For this review, take the finished solid that the model builds, in its own axes (mm). Face numbers are marked on the shaded views. A direction names the side the tool comes from. Coordinates: 2 decimals unless noted, no trailing zeros. Write each loop counter-clockwise with the first axis right and the second up, starting at its lowest first coordinate (ties: lowest second). Pieces come first, ordered by that corner, then holes. Notation, with made-up numbers: (52, 10) - (87, 10) arc R27 ccw to (87, 46) - close; hole circle Ø6 at (41, 44.25). An arc over 180 degrees is marked (long way). Use one line per item in the form item = value. Start each with the question number.
1) We need section C-C (x = 20). Give the boundary of the cut face in (y, z), plus the area to 3 significant figures.
2) Mouldability with a two-part tool opening along X and no side actions: class the marked faces 1, 2 and 3 as pulls with the +X half, pulls with the -X half, needs draft (parallel to the pull), parting line crosses it, or undercut.
3) We need section B-B (x = -22). Give the boundary of the cut face in (y, z).
4) We need section D-D (y = -24). Give the boundary of the cut face in (x, z), plus the area to 3 significant figures.
5) Tool access review of the marked faces 4 and 5: name each direction out of +Z, -Z, +X, -X, +Y, -Y from which nothing blocks a thin tool from reaching the whole face with its end or side.
6) Insertion check: P1, Ø6, axis at y = 11.5, z = 35, coming from the -X side (3 decimals); P2, Ø10, axis at y = 10, z = 96, coming from the -X side; P3, Ø4.5, axis at x = 0, y = 0, coming from the +Z side; P4, Ø10, axis at x = -18, y = 18, coming from the +Z side. Each pin has a flat end and moves straight along its axis. Give the tip position at first contact, or say it passes through.
7) For L1, parallel to X at y = -4, z = 90.5; L2, parallel to X at y = 0, z = 7.25; L3, parallel to X at y = -34.5, z = 57, list the stretches that pass through material, from the lowest coordinate up. Write a range as from..to.
```python
from build123d import *

# Parameters (mm, degrees)
SKETCH1_R           = 6.35
BOSS_EXTRUDE5_DEPTH = 220
SKETCH9_R           = 10
BOSS_EXTRUDE6_DEPTH = 2.5
SKETCH10_R          = 12.5
BOSS_EXTRUDE7_DEPTH = 2
SKETCH7_R           = 2.54
CUT_EXTRUDE1_DEPTH  = 19
CUT_EXTRUDE2_DEPTH  = 19


with BuildPart() as part:
    # Sketch1 → Boss-Extrude5 (new body)
    with BuildSketch(Plane.XY):
        Circle(SKETCH1_R)
        with BuildLine():
            ThreePointArc((0.744012112, -6.306262441), (0.372648292, -6.33905618), (0, -6.35))
            Line((0, -6.35), (0, -38.1))
            ThreePointArc((0, -38.1), (2.307620454, -36.88268092), (3.706666044, -34.680488981))
            ThreePointArc((3.706666044, -34.680488981), (3.812853299, -34.161384534), (3.809033576, -33.631544397))
            Line((3.809033576, -33.631544397), (0.744012112, -6.306262441))
        make_face()
        with BuildLine():
            ThreePointArc((-5.089377421, -3.79746461), (-5.303459542, -3.492250977), (-5.499261314, -3.175))
            Line((-5.499261314, -3.175), (-32.995567884, -19.05))
            ThreePointArc((-32.995567884, -19.05), (-30.78752841, -20.439798395), (-28.180851452, -20.550311448))
            ThreePointArc((-28.180851452, -20.550311448), (-27.678200185, -20.382720085), (-27.221255028, -20.114492039))
            Line((-27.221255028, -20.114492039), (-5.089377421, -3.79746461))
        make_face()
        with BuildLine():
            ThreePointArc((-5.833389533, 2.508797831), (-5.676107834, 2.846805203), (-5.499261314, 3.175))
            Line((-5.499261314, 3.175), (-32.995567884, 19.05))
            ThreePointArc((-32.995567884, 19.05), (-33.095148863, 16.442882525), (-31.887517495, 14.130177533))
            ThreePointArc((-31.887517495, 14.130177533), (-31.491053484, 13.778664449), (-31.030288604, 13.517052358))
            Line((-31.030288604, 13.517052358), (-5.833389533, 2.508797831))
        make_face()
        with BuildLine():
            Line((-3.809033576, 33.631544397), (-0.744012112, 6.306262441))
            ThreePointArc((-0.744012112, 6.306262441), (-0.372648292, 6.33905618), (0, 6.35))
            Line((0, 6.35), (0, 38.1))
            ThreePointArc((0, 38.1), (-2.307620454, 36.88268092), (-3.706666044, 34.680488981))
            ThreePointArc((-3.706666044, 34.680488981), (-3.812853299, 34.161384534), (-3.809033576, 33.631544397))
        make_face()
        with BuildLine():
            Line((27.221255028, 20.114492039), (5.089377421, 3.79746461))
            ThreePointArc((5.089377421, 3.79746461), (5.303459542, 3.492250977), (5.499261314, 3.175))
            Line((5.499261314, 3.175), (32.995567884, 19.05))
            ThreePointArc((32.995567884, 19.05), (30.78752841, 20.439798395), (28.180851452, 20.550311448))
            ThreePointArc((28.180851452, 20.550311448), (27.678200185, 20.382720085), (27.221255028, 20.114492039))
        make_face()
        with BuildLine():
            Line((31.030288604, -13.517052358), (5.833389533, -2.508797831))
            ThreePointArc((5.833389533, -2.508797831), (5.676107834, -2.846805203), (5.499261314, -3.175))
            Line((5.499261314, -3.175), (32.995567884, -19.05))
            ThreePointArc((32.995567884, -19.05), (33.095148863, -16.442882525), (31.887517495, -14.130177533))
            ThreePointArc((31.887517495, -14.130177533), (31.491053484, -13.778664449), (31.030288604, -13.517052358))
        make_face()
    extrude(amount=BOSS_EXTRUDE5_DEPTH)

    # Sketch9 → Boss-Extrude6 (add)
    with BuildSketch(Plane(origin=(0, 0, 0), x_dir=(-1, 0, 0), z_dir=(0, 0, -1))):
        with Locations(Location((0, 0, 0), (0, 0, 203.391310961))):
            Circle(SKETCH9_R)
    extrude(amount=BOSS_EXTRUDE6_DEPTH)

    # Sketch10 → Boss-Extrude7 (add)
    with BuildSketch(Plane(origin=(0, 0, -2.5), x_dir=(-1, 0, 0), z_dir=(0, 0, -1))):
        Circle(SKETCH10_R)
    extrude(amount=BOSS_EXTRUDE7_DEPTH)

    # Sketch7 → Cut-Extrude1 (cut)
    with BuildSketch(Plane.XY.offset(220)):
        Circle(SKETCH7_R)
    extrude(amount=-CUT_EXTRUDE1_DEPTH, mode=Mode.SUBTRACT)

    # Sketch11 → Cut-Extrude2 (cut)
    with BuildSketch(Plane(origin=(0, 0, -4.5), x_dir=(-1, 0, 0), z_dir=(0, 0, -1))):
        with BuildLine():
            Line((-1.12, 1.042353107), (1.12, 1.042353107))
            ThreePointArc((1.12, 1.042353107), (0, -1.53), (-1.12, 1.042353107))
        make_face()
    extrude(amount=-CUT_EXTRUDE2_DEPTH, mode=Mode.SUBTRACT)


solid = part.part
```
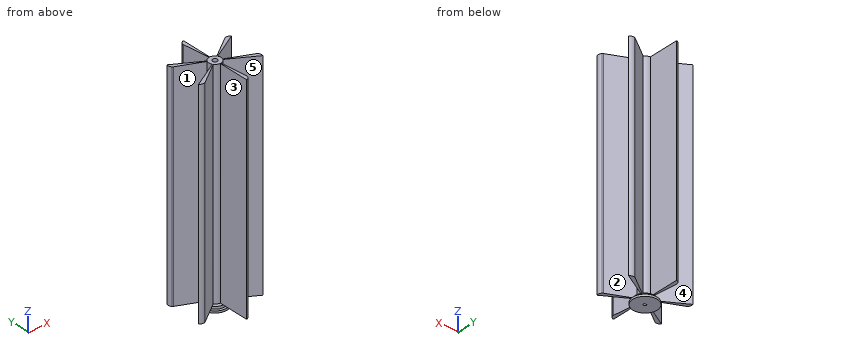
Determined:
q1.outline = (-11.55, 0) - (-8.7, 0) - (-8.7, 220) - (-11.55, 220) - close; (11.55, 0) - (14.79, 0) - (14.79, 220) - (11.55, 220) - close
q1.area = 1,340 mm²
q2.face_1 = pulls with the -X half
q2.face_2 = pulls with the +X half
q2.face_3 = undercut
q3.outline = (-16.27, 0) - (-12.7, 0) - (-12.7, 220) - (-16.27, 220) - close; (9.57, 0) - (12.7, 0) - (12.7, 220) - (9.57, 220) - close
q4.outline = (0, 0) - (2.73, 0) - (2.73, 220) - (0, 220) - close
q4.area = 600 mm²
q5.face_4 = +Z, +Y
q5.face_5 = +Z, -Y
q6.P1 = -32.195
q6.P2 = -32.53
q6.P3 = 201
q6.P4 = through
q7.L1 = -6.93..-5.36, -4.93..4.93, 6.93..9.25
q7.L2 = -6.35..-1.53, 1.53..6.35
q7.L3 = 0..3.76
